from build123d import *

# Parameters (mm, degrees)
BOSS_EXTRUDE1_DEPTH      = 110
SKETCH2_R                = 3
CUT_EXTRUDE1_DEPTH       = 55
BOSS_EXTRUDE2_DEPTH      = 114
BOSS_EXTRUDE2_DEPTH_BACK = 4
FILLET1_R                = 2


with BuildPart() as part:
    # Sketch1 → Boss-Extrude1 (new body)
    # profile 1 of 2: a face of its own
    with BuildSketch(Plane.XY):
        with BuildLine():
            ThreePointArc((41.937258351, 46.258124568), (38.471168757, 49.184002684), (34.802002476, 51.850790754))
            Line((34.802002476, 51.850790754), (21.730642096, 38.779430374))
            ThreePointArc((21.730642096, 38.779430374), (31.38159768, 31.459823211), (38.701204844, 21.808867626))
            Line((38.701204844, 21.808867626), (51.772565224, 34.880228006))
            ThreePointArc((51.772565224, 34.880228006), (49.105777153, 38.549394287), (46.179899038, 42.015483881))
            Line((46.179899038, 42.015483881), (39.099113563, 34.934698406))
            Line((39.099113563, 34.934698406), (34.856472876, 39.177339093))
            Line((34.856472876, 39.177339093), (41.937258351, 46.258124568))
        make_face()
        Polygon((27.431851673, 38.116678921), (30.260278798, 40.945106046), (40.866880516, 30.338504328), (38.038453391, 27.510077204), align=None, mode=Mode.SUBTRACT)
    # profile 2 of 2: a face of its own
    with BuildSketch(Plane.XY):
        Polygon((38.038453391, 27.510077204), (40.866880516, 30.338504328), (30.260278798, 40.945106046), (27.431851673, 38.116678921), align=None)
    extrude(amount=BOSS_EXTRUDE1_DEPTH)

    # Sketch2 → Cut-Extrude1 (cut, symmetric)
    with BuildSketch(Plane(origin=(2.082207578, -2.082207578, 0), x_dir=(0, 0, 1), z_dir=(-0.7071067811865467, 0.7071067811865485, 0))):
        with Locations(Location((85, 57.356681906, 0), (0, 0, 90))):
            Circle(SKETCH2_R)
        with Locations(Location((55, 57.356681906, 0), (0, 0, 90))):
            Circle(SKETCH2_R)
        with Locations(Location((25, 57.356681906, 0), (0, 0, 90))):
            Circle(SKETCH2_R)
    extrude(amount=CUT_EXTRUDE1_DEPTH, both=True, mode=Mode.SUBTRACT)

    # Sketch1_5 → Boss-Extrude2 (add, two sides: drawn at the far end of the back side and taken through both)
    with BuildSketch(Plane.XY.offset(-BOSS_EXTRUDE2_DEPTH_BACK)):
        Polygon((38.038453391, 27.510077204), (40.866880516, 30.338504328), (30.260278798, 40.945106046), (27.431851673, 38.116678921), align=None)
    extrude(amount=BOSS_EXTRUDE2_DEPTH + BOSS_EXTRUDE2_DEPTH_BACK)

    # Fillet1
    fillet1_edges = [part.edges().sort_by_distance(p)[0] for p in [
        (39.452666954, 28.924290766, -4),
        (28.846065236, 39.530892484, -4),
        (39.452666954, 28.924290766, 114),
        (28.846065236, 39.530892484, 114),
    ]]
    fillet(fillet1_edges, radius=FILLET1_R)


solid = part.part
The model under review builds one solid part; all positions refer to its coordinate system, in mm. A direction names the side the tool comes from. Coordinates: 2 decimals unless noted, no trailing zeros. Write each loop counter-clockwise with the first axis right and the second up, starting at its lowest first coordinate (ties: lowest second). Pieces come first, ordered by that corner, then holes. Notation, with made-up numbers: (-21.75, 79.25) -> (-0.75, 79.25) arc R11 cw to (-0.75, 93.25) -> close; hole circle Ø4 at (15.5, 84.25). An arc over 180 degrees is marked (long way). Answer in a Markdown table with one row per item.
1. Clearance check with flat-ended pins moving along their axes: pin 1 Ø1.5 at (y, z) = (39.5, 78.5) entering from +X; pin 2 Ø6 at (x, y) = (29, 29.5) entering from -Z; pin 3 Ø1.5 at (y, z) = (46.5, 17) entering from +X; pin 4 Ø1 at (y, z) = (34.5, 38.5) entering from -X. State where each tip first meets the part, or that it passes through.
Answers below:
| item | result |
|---|---|
| pin 1 | stops at x = 48.95 |
| pin 2 | passes through |
| pin 3 | stops at x = 41.94 |
| pin 4 | stops at x = 27.39 |
2. We need section B-B, the plane x = 25. State the section outline as (y, z) points, and give its area (3 significant figures).
Answers below:
| item | result |
|---|---|
| outline | (36.75, 0) -> (42.05, 0) -> (42.05, 110) -> (36.75, 110) -> close |
| area | 583 mm^2 |
3. Draft analysis for pull direction X (two halves, no side actions). For faces 4 (the flat face through (37.8, 35.8, 0)), 5 (the flat face through (39.43, 28.9, -1.01)), 6 (the flat face through (40.329, 36.164, 54.23)), state which applies: +X half, -X half, draft (parallel to the pull), parting line (faces both ways), or undercut.
Answers below:
| item | result |
|---|---|
| face 4 | draft |
| face 5 | +X half |
| face 6 | undercut |
4. For faces 1 (the flat face through (32.66, 32.89, -2.03)), 2 (the flat face through (28.866, 39.551, 110.986)), 3 (the flat face through (39.43, 28.9, 110.99)), list the 3-axis set-ups (+Z, -Z, +X, -X, +Y, -Y) from which the entire face can be reached by the end or side of a thin tool; tool diameter is ignored.
Answers below:
| item | result |
|---|---|
| face 1 | -Z, -X, -Y |
| face 2 | +Z, -X, +Y |
| face 3 | +Z, +X, -Y |
5. We need section C-C, the plane y = 24. State the section outline as (x, z) points.
Answers below:
| item | result |
|---|---|
| outline | (37.38, 0) -> (40.89, 0) -> (40.89, 110) -> (37.38, 110) -> close |
6. Wall thickness on probe 1 along Z at (x, y) = (35.5, 46); probe 2 along Z at (x, y) = (35, 50); probe 3 along X at (y, z) = (38.5, 10): over which ranges is each line inside the solid? List them lowest first. Write a range as [from, to].
Answers below:
| item | result |
|---|---|
| probe 1 | z = [0, 22.01], [27.99, 52.01], [57.99, 82.01], [87.99, 110] |
| probe 2 | z = [0, 23.8], [26.2, 53.8], [56.2, 83.8], [86.2, 110] |
| probe 3 | x = [22.22, 35.53], [42.66, 49.14] |
7. We need section A-A, the plane z = 39. State the section outline as (x, y) points.
Answers below:
| item | result |
|---|---|
| outline | (21.73, 38.78) arc R44.5 cw to (38.7, 21.81) -> (51.77, 34.88) arc R62.5 ccw to (46.18, 42.02) -> (39.1, 34.93) -> (34.86, 39.18) -> (41.94, 46.26) arc R62.5 ccw to (34.8, 51.85) -> close |
